```python
from build123d import *

# Parameters (mm, degrees)
SKETCH1_W           = 135
SKETCH1_H           = 12.93762629
BOSS_EXTRUDE1_DEPTH = 9
SKETCH2_W           = 7
SKETCH2_H           = 12.93762629
BOSS_EXTRUDE2_DEPTH = 54
SKETCH3_W           = 7
SKETCH3_H           = 12.93762629
BOSS_EXTRUDE5_DEPTH = 13
BOSS_EXTRUDE6_REACH = 129.212
SKETCH6_W           = 30
SKETCH6_H           = 12.93762629
SKETCH7_R           = 1.5
CUT_EXTRUDE1_DEPTH  = 5
SKETCH9_W           = 25
SKETCH9_H           = 3.5
BOSS_EXTRUDE7_DEPTH = 5.5
CUT_EXTRUDE3_DEPTH  = 9


with BuildPart() as part:
    # Sketch1 → Boss-Extrude1 (new body)
    with BuildSketch(Plane.XY):
        with Locations((60, 0)):
            Rectangle(SKETCH1_W, SKETCH1_H)
    extrude(amount=BOSS_EXTRUDE1_DEPTH)

    # Sketch2 → Boss-Extrude2 (add)
    with BuildSketch(Plane(origin=(0, 0, 0), x_dir=(-1, 0, 0), z_dir=(0, 0, -1))):
        with Locations((-124, 0)):
            Rectangle(SKETCH2_W, SKETCH2_H)
    extrude(amount=BOSS_EXTRUDE2_DEPTH)

    # Sketch3 → Boss-Extrude5 (add)
    with BuildSketch(Plane.ZY.offset(-120.5)):
        with Locations((-50.5, 0)):
            Rectangle(SKETCH3_W, SKETCH3_H)
    extrude(amount=BOSS_EXTRUDE5_DEPTH)

    # Boss-Extrude6: up to this face of the body (flat: up to its plane)
    boss_extrude6_end = Plane(part.part.faces().sort_by_distance((127.5, 0, -22.5))[0])
    # Sketch6 → Boss-Extrude6 (add, up to the picked face)
    with BuildSketch(Plane.ZY.offset(-107.5), mode=Mode.PRIVATE) as boss_extrude6_sk1:
        with Locations((-52, 0)):
            Rectangle(SKETCH6_W, SKETCH6_H)
    boss_extrude6_tool1 = split(extrude(boss_extrude6_sk1.sketch, amount=-BOSS_EXTRUDE6_REACH, mode=Mode.PRIVATE), bisect_by=boss_extrude6_end, keep=Keep.BOTH, mode=Mode.PRIVATE)
    add(boss_extrude6_tool1.solids().sort_by(Axis((107.5, 0, -52), (1, 0, 0)))[0])

    # Sketch7 → Cut-Extrude1 (cut)
    with BuildSketch(Plane.ZY.offset(-107.5)):
        with Locations((-39.75, -3.718813145)):
            Circle(SKETCH7_R)
        with Locations((-58.8, -3.718813145)):
            Circle(SKETCH7_R)
    extrude(amount=-CUT_EXTRUDE1_DEPTH, mode=Mode.SUBTRACT)

    # Sketch9 → Boss-Extrude7 (add)
    with BuildSketch(Plane.ZY.offset(-107.5)):
        with Locations((-49.5, 4.718813145)):
            Rectangle(SKETCH9_W, SKETCH9_H)
    extrude(amount=BOSS_EXTRUDE7_DEPTH)

    # Sketch12 → Cut-Extrude3 (cut)
    with BuildSketch(Plane.XY.offset(9)):
        with BuildLine():
            Line((-1, 2.75), (9, 2.75))
            ThreePointArc((9, 2.75), (11.75, 0), (9, -2.75))
            Line((9, -2.75), (-1, -2.75))
            ThreePointArc((-1, -2.75), (-3.75, 0), (-1, 2.75))
        make_face()
        with BuildLine():
            Line((109, -2.75), (99, -2.75))
            ThreePointArc((99, -2.75), (96.25, 0), (99, 2.75))
            Line((99, 2.75), (109, 2.75))
            ThreePointArc((109, 2.75), (111.75, 0), (109, -2.75))
        make_face()
    extrude(amount=-CUT_EXTRUDE3_DEPTH, mode=Mode.SUBTRACT)


solid = part.part
```
Could you check a few things on this model? Use its own coordinates, in mm. A direction names the side the tool comes from. Round coordinates to 2 decimals unless told otherwise and drop trailing zeros. Loops run counter-clockwise (first coordinate to the right, second up) from the corner with the lowest first, then second, coordinate; pieces in that order, holes last. Notation, with made-up numbers: (81.5, -19) - (98.5, -19) arc R22 cw to (98.5, 13) - close; hole circle Ø10 at (59.25, 2.25). An arc over 180 degrees is marked (long way). Answer in a Markdown table with one row per item. Add a question column.
(1) If we mould it in two halves opening along Z, with no side actions, what happens to faces 4 (the face through (112.5, -4, -59)), 5 (the face through (105, 5, -62)), 6 (the face through (112.5, -4, -40)), 7 (the face through (127.5, 0, -28))? For each: pulls with the +Z half, pulls with the -Z half, needs draft (parallel to the pull), parting line crosses it, or undercut.
(2) If we section it at B-B (z = -39.75): Please give me the cut outline in (x, y), plus the area to 3 significant figures.
(3) If we section it at A-A (y = 0): Please give me the cut outline in (x, z), plus the area to 4 significant figures.
(4) I'm going to push flat-ended pins straight in: pin 1 (1.5 mm diameter, centred on y = -3, z = -27, fed in from -X); pin 2 (0.9 mm diameter, centred on y = -3.5, z = -59, fed in from -X); pin 3 (3 mm diameter, centred on x = 103.5, y = 4.5, fed in from -Z). Where does each tip first touch, or does it pass through?
(5) If we section it at C-C (x = 57): Please give me the cut outline in (y, z).
(6) If we section it at D-D (z = -20): Please give me the cut outline in (x, y).
(7) For faces 1 (the face through (11.75, 0.06, 4.56)), 2 (the face through (105, 2.969, -50)), 3 (the face through (113, 0, -37)), which set-ups out of +Z, -Z, +X, -X, +Y, -Y let a thin tool reach every point of the face, with its end or its side?
(8) I need wall thicknesses on line 1 along Z through (x, y) = (118.5, -1); line 2 along Y through (x, z) = (111.2, -58.8); line 3 along Z through (x, y) = (24, 5.5). Which ranges of each line are inside material? Lowest first, please.
Model answer:
| question | item | result |
|---|---|---|
| 1 | face 4 | undercut |
| 1 | face 5 | pulls with the -Z half |
| 1 | face 6 | undercut |
| 1 | face 7 | needs draft |
| 2 | outline | (102, 2.97) - (107.5, 2.97) - (107.5, -2.22) - (112.5, -2.22) - (112.5, -5.22) - (107.5, -5.22) - (107.5, -6.47) - (127.5, -6.47) - (127.5, 6.47) - (102, 6.47) - close |
| 2 | area | 263 mm² |
| 3 | outline | (-7.5, 0) - (-3.75, 0) - (-3.75, 9) - (-7.5, 9) - close; (11.75, 0) - (96.25, 0) - (96.25, 9) - (11.75, 9) - close; (107.5, -67) - (127.5, -67) - (127.5, 9) - (111.75, 9) - (111.75, 0) - (120.5, 0) - (120.5, -37) - (107.5, -37) - close |
| 3 | area | 1,795 mm² |
| 4 | pin 1 | stops at x = 120.5 |
| 4 | pin 2 | stops at x = 112.5 |
| 4 | pin 3 | stops at z = -62 |
| 5 | outline | (-6.47, 0) - (6.47, 0) - (6.47, 9) - (-6.47, 9) - close |
| 6 | outline | (120.5, -6.47) - (127.5, -6.47) - (127.5, 6.47) - (120.5, 6.47) - close |
| 7 | face 1 | +Z, -Z |
| 7 | face 2 | -Z, -X, -Y |
| 7 | face 3 | -X, +Y, -Y |
| 8 | line 1 | z = -67 to -37, 0 to 9 |
| 8 | line 2 | y = -6.47 to -5.22, -2.22 to 6.47 |
| 8 | line 3 | z = 0 to 9 |
